Geometry: final body of the model. Coordinates: model frame, mm. Face numbers are marked on the shaded views. A direction names the side the tool comes from. Give positions to 0.01 mm unless a question says otherwise; leave off trailing zeros. Order: outer loops, then holes, each group sorted by start corner. A loop starts at its lowest first (then second) coordinate and runs counter-clockwise, first axis right, second up. Notation, with made-up numbers: (-0.5, 29) - (22.5, 29) arc R23 cw to (22.5, 40) - close; hole circle Ø5 at (65.5, -8). An arc over 180 degrees is marked (long way). One line per item, written item: value.
```python
from build123d import *

# Parameters (mm, degrees)
SKETCH_W        = 40
SKETCH_H        = 30
PAD_DEPTH       = 8
SKETCH001_R     = 1
SKETCH001_W     = 33.6
SKETCH001_H     = 25
POCKET_DEPTH    = 5
SKETCH002_R     = 1
POCKET001_DEPTH = 3.2
POCKET002_DEPTH = 3.2
SKETCH003_R     = 1
POCKET003_DEPTH = 2
SKETCH004_R     = 1
POCKET004_DEPTH = 2
FILLET_R        = 0.5
SKETCH005_R     = 1
POCKET005_DEPTH = 3.2


with BuildPart() as part:
    # Sketch (on Sketch) → Pad (new body)
    with BuildSketch(Plane.XY):
        Rectangle(SKETCH_W, SKETCH_H)
    extrude(amount=PAD_DEPTH)

    # Sketch001 (on Face6 of Pad) → Pocket (cut)
    with BuildSketch(Plane.XY.offset(8)):
        with Locations((-18.4, 13.75)):
            Circle(SKETCH001_R)
        with Locations((-6.4, 13.75)):
            Circle(SKETCH001_R)
        with Locations((6.4, 13.75)):
            Circle(SKETCH001_R)
        with Locations((18.4, 13.75)):
            Circle(SKETCH001_R)
        with Locations((-18.4, -13.75)):
            Circle(SKETCH001_R)
        with Locations((-6.4, -13.75)):
            Circle(SKETCH001_R)
        with Locations((6.4, -13.75)):
            Circle(SKETCH001_R)
        with Locations((18.4, -13.75)):
            Circle(SKETCH001_R)
        Rectangle(SKETCH001_W, SKETCH001_H)
    extrude(amount=-POCKET_DEPTH, mode=Mode.SUBTRACT)

    # Sketch002 (on Face2 of Pocket) → Pocket001 (cut)
    with BuildSketch(Plane(origin=(-20, 0, 0), x_dir=(0, -1, 0), z_dir=(-1, 0, 0))):
        with Locations((-6.15, 3.3)):
            Circle(SKETCH002_R)
        with Locations((6.15, 3.3)):
            Circle(SKETCH002_R)
        with Locations((0, 3.3)):
            Circle(SKETCH002_R)
    extrude(amount=-POCKET001_DEPTH, mode=Mode.SUBTRACT)

    # Sketch002 (on Face2 of Pocket) → Pocket002 (cut)
    with BuildSketch(Plane(origin=(-20, 0, 0), x_dir=(0, -1, 0), z_dir=(-1, 0, 0))):
        with Locations((-6.15, 3.3)):
            Circle(SKETCH002_R)
        with Locations((6.15, 3.3)):
            Circle(SKETCH002_R)
        with Locations((0, 3.3)):
            Circle(SKETCH002_R)
    extrude(amount=-POCKET002_DEPTH, mode=Mode.SUBTRACT)

    # Sketch003 → Pocket003 (cut)
    with BuildSketch(Plane.XY.offset(5)):
        with Locations((-12, 10)):
            Circle(SKETCH003_R)
        with Locations((12, 10)):
            Circle(SKETCH003_R)
        with Locations((12, -10)):
            Circle(SKETCH003_R)
        with Locations((-12, -10)):
            Circle(SKETCH003_R)
    extrude(amount=-POCKET003_DEPTH, mode=Mode.SUBTRACT)

    # Sketch004 (on Face4 of Pocket003) → Pocket004 (cut)
    with BuildSketch(Plane(origin=(0, 0, 0), x_dir=(1, 0, 0), z_dir=(0, 0, -1))):
        with Locations((-10, 5)):
            Circle(SKETCH004_R)
        with Locations((0, 5)):
            Circle(SKETCH004_R)
        with Locations((10, 5)):
            Circle(SKETCH004_R)
        with Locations((10, -5)):
            Circle(SKETCH004_R)
        with Locations((0, -5)):
            Circle(SKETCH004_R)
        with Locations((-10, -5)):
            Circle(SKETCH004_R)
    extrude(amount=-POCKET004_DEPTH, mode=Mode.SUBTRACT)

    # Fillet
    fillet_edges = [part.edges().sort_by_distance(p)[0] for p in [
        (20, -15, 4),
        (-16.8, 12.5, 5.5),
        (-20, -15, 4),
        (-20, 15, 4),
        (-16.8, -12.5, 5.5),
        (16.8, 12.5, 5.5),
        (16.8, -12.5, 5.5),
        (20, 15, 4),
    ]]
    fillet(fillet_edges, radius=FILLET_R)

    # Sketch005 (on Face7 of Fillet) → Pocket005 (cut)
    with BuildSketch(Plane.YZ.offset(20)):
        with Locations((-6.15, 3.3)):
            Circle(SKETCH005_R)
        with Locations((6.15, 3.3)):
            Circle(SKETCH005_R)
        with Locations((0, 3.3)):
            Circle(SKETCH005_R)
    extrude(amount=-POCKET005_DEPTH, mode=Mode.SUBTRACT)


solid = part.part
```
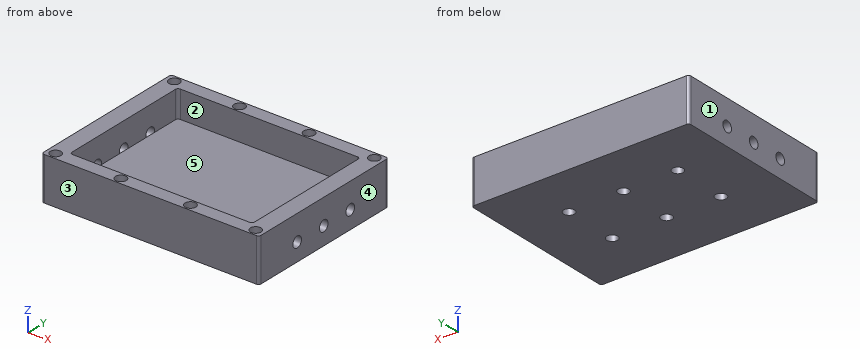
1) Material intervals for line 1 along Y through (x, z) = (-6.4, 5.75); line 2 along Y through (x, z) = (-18.4, 6.8); line 3 along X through (y, z) = (1.75, 5.25), sorted ascending.
Answers below:
line 1: -15 to -14.75, -12.75 to -12.5, 12.5 to 12.75, 14.75 to 15
line 2: -15 to -14.75, -12.75 to 12.75, 14.75 to 15
line 3: -20 to -16.8, 16.8 to 20
2) Section A-A, the plane y = 0. Return loops of the section in (x, z).
Answers below:
outline: (-20, 0) - (20, 0) - (20, 2.3) - (16.8, 2.3) - (16.8, 3) - (-16.8, 3) - (-16.8, 2.3) - (-20, 2.3) - close; (-20, 4.3) - (-16.8, 4.3) - (-16.8, 8) - (-20, 8) - close; (16.8, 4.3) - (20, 4.3) - (20, 8) - (16.8, 8) - close
3) Section C-C, the plane x = 3. Return loops of the section in (y, z), then the cut area to 3 significant figures.
Answers below:
outline: (-15, 0) - (15, 0) - (15, 8) - (12.5, 8) - (12.5, 3) - (-12.5, 3) - (-12.5, 8) - (-15, 8) - close
area: 115 mm^2
4) First-contact query: pin 1 (2.5 mm diameter, centred on x = -6.4, y = 13.75, fed in from -Z); pin 2 (1.8 mm diameter, centred on x = -10, y = -5, fed in from +Z). Flat tips, straight axial feed; report the tip coordinate or a pass-through.
Answers below:
pin 1: z = 0
pin 2: z = 3
5) Set-up query: the marked faces 1 and 2. Return all of +Z, -Z, +X, -X, +Y, -Y with unobstructed straight access to the full face (end or side cutting, diameter ignored); none if empty.
Answers below:
face 1: +Z, -Z, -X, +Y, -Y
face 2: +Z
6) Section D-D, the plane y = 3.5. Return loops of the section in (x, z).
Answers below:
outline: (-20, 0) - (20, 0) - (20, 8) - (16.8, 8) - (16.8, 3) - (-16.8, 3) - (-16.8, 8) - (-20, 8) - close
7) Mould query, pull axis Y, two halves, no side actions, for the marked faces 3, 4 and 5. Classes: released by +Y, released by -Y, zero draft, split by the parting line, or undercut.
Answers below:
face 3: released by -Y
face 4: zero draft
face 5: undercut
8) Section B-B, the plane z = 5. Count the separate pieces of the cut face and the enclosed holes in it, then the cut area to 3 significant figures.
Answers below:
separate pieces: 1
enclosed holes: 9
area: 335 mm^2
